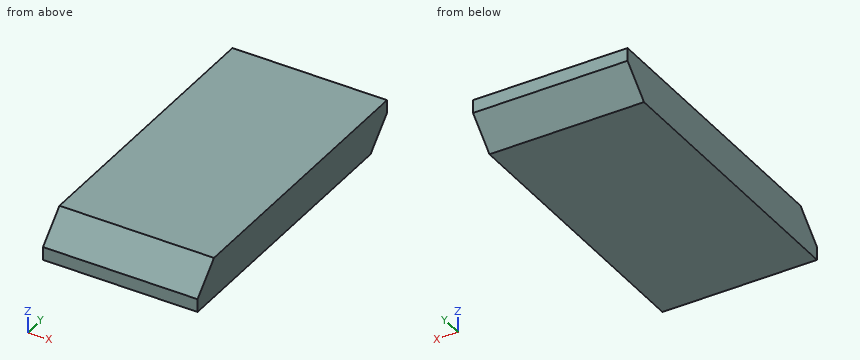
```python
from build123d import *

# Parameters (mm, degrees)
SKETCH1_W           = 25.4
SKETCH1_H           = 51.181
BOSS_EXTRUDE1_DEPTH = 6.604
CHAMFER1_SIZE       = 4.445


with BuildPart() as part:
    # Sketch1 → Boss-Extrude1 (new body)
    with BuildSketch(Plane.XY):
        with Locations((0, -47.625)):
            Rectangle(SKETCH1_W, SKETCH1_H)
    extrude(amount=BOSS_EXTRUDE1_DEPTH)

    # Chamfer1
    chamfer1_edges = [part.edges().sort_by_distance(p)[0] for p in [
        (0, -73.2155, 6.604),
        (0, -22.0345, 0),
    ]]
    chamfer(chamfer1_edges, length=CHAMFER1_SIZE)


solid = part.part
```
Work out the finished part from the listing and answer in its coordinate system (mm). Round coordinates to 2 decimals unless told otherwise and drop trailing zeros. Write each loop counter-clockwise with the first axis right and the second up, starting at its lowest first coordinate (ties: lowest second). Pieces come first, ordered by that corner, then holes. Notation, with made-up numbers: (25.25, 72.25) -> (80.25, 72.25) arc R14 ccw to (80.25, 82.25) -> close; hole circle Ø1 at (-20, -36.5). An arc over 180 degrees is marked (long way). Write each question's results on one line, items separated by ' | '.
Q1. Straight lines are drawn through the part: line 1 along Y through (x, z) = (-6.5, 3.75); line 2 along Y through (x, z) = (-6, 5.5); line 3 along Z through (x, y) = (-3.25, -69.5). For each, find the intervals that lie inside material, in ascending order. Write a range as [from, to].
Data:
line 1: [-71.62, -22.73] | line 2: [-69.87, -22.03] | line 3: [0, 5.87]
Q2. Section B-B, the plane z = 5.5 is taken. Write down the section's boundary in (x, y).
Data:
outline: (-12.7, -69.87) -> (12.7, -69.87) -> (12.7, -22.03) -> (-12.7, -22.03) -> close
Q3. A flat-ended cylindrical pin translates along its axis: P1, Ø1.5, axis at x = -9.5, z = 6, coming from the -Y side. Find the tip coordinate at first contact, or state that the pin passes through.
Data:
P1: y = -70.12
Q4. Section C-C, the plane y = -26 is taken. Write down the section's boundary in (x, z).
Data:
outline: (-12.7, 0.48) -> (12.7, 0.48) -> (12.7, 6.6) -> (-12.7, 6.6) -> close
Q5. Section A-A, the plane x = -10.5 is taken. Write down the section's boundary in (y, z) (1 decimal), then the cut area to 3 significant figures.
Data:
outline: (-73.2, 0) -> (-26.5, 0) -> (-22, 4.4) -> (-22, 6.6) -> (-68.8, 6.6) -> (-73.2, 2.2) -> close | area: 318 mm^2
